```python
from build123d import *

# Parameters (mm, degrees)
SCHIZZO1_W                   = 180
SCHIZZO1_H                   = 60
ESTRUSIONE_ESTRUSIONE1_DEPTH = 5
SCHIZZO1_3_W                 = 180
SCHIZZO1_3_H                 = 10
ESTRUSIONE_ESTRUSIONE2_DEPTH = 100
SCHIZZO2_W                   = 180
SCHIZZO2_H                   = 5
ESTRUSIONE_ESTRUSIONE3_DEPTH = 60
SCHIZZO3_W                   = 5
SCHIZZO3_H                   = 90
ESTRUSIONE_ESTRUSIONE4_DEPTH = 60
SCHIZZO4_W                   = 12
SCHIZZO4_H                   = 3
TAGLIO_ESTRUSIONE1_DEPTH     = 90
SCHIZZO6_W                   = 2
SCHIZZO6_H                   = 15.540639337
ESTRUSIONE_ESTRUSIONE5_DEPTH = 10
SCHIZZO10_W                  = 16
SCHIZZO10_H                  = 3
ESTRUSIONE_ESTRUSIONE7_DEPTH = 30
SCHIZZO11_W                  = 12
SCHIZZO11_H                  = 3
TAGLIO_ESTRUSIONE6_DEPTH     = 5
SCHIZZO12_W                  = 9
SCHIZZO12_H                  = 3
TAGLIO_ESTRUSIONE7_DEPTH     = 20
SCHIZZO13_W                  = 2
SCHIZZO13_H                  = 35.114164676
ESTRUSIONE_ESTRUSIONE8_DEPTH = 10
TAGLIO_ESTRUSIONE8_START     = -15.540639
SCHIZZO15_W                  = 21.926890516
SCHIZZO15_H                  = 11.981890919
TAGLIO_ESTRUSIONE8_DEPTH     = 15.540639
SCHIZZO16_W                  = 12
SCHIZZO16_H                  = 3
ESTRUSIONE_ESTRUSIONE9_DEPTH = 5
SCHIZZO17_R                  = 9.5
TAGLIO_ESTRUSIONE9_DEPTH     = 6
SCHIZZO21_W                  = 2
SCHIZZO21_H                  = 50
TAGLIO_ESTRUSIONE10_DEPTH    = 2


with BuildPart() as part:
    # Schizzo1 → Estrusione-Estrusione1 (new body)
    with BuildSketch(Plane(origin=(0, 0, 0), x_dir=(1, 0, 0), z_dir=(0, 1, 0))):
        with Locations((90, 30)):
            Rectangle(SCHIZZO1_W, SCHIZZO1_H)
    extrude(amount=ESTRUSIONE_ESTRUSIONE1_DEPTH)

    # Schizzo1<3> → Estrusione-Estrusione2 (add)
    with BuildSketch(Plane(origin=(0, 0, 0), x_dir=(1, 0, 0), z_dir=(0, 1, 0))):
        with Locations((90, 65)):
            Rectangle(SCHIZZO1_3_W, SCHIZZO1_3_H)
    extrude(amount=ESTRUSIONE_ESTRUSIONE2_DEPTH)

    # Schizzo2 → Estrusione-Estrusione3 (add)
    with BuildSketch(Plane.XY.offset(-60)):
        with Locations((90, 97.5)):
            Rectangle(SCHIZZO2_W, SCHIZZO2_H)
    extrude(amount=ESTRUSIONE_ESTRUSIONE3_DEPTH)

    # Schizzo3 → Estrusione-Estrusione4 (add)
    with BuildSketch(Plane.XY.offset(-60)):
        with Locations((2.5, 50)):
            Rectangle(SCHIZZO3_W, SCHIZZO3_H)
        with Locations((177.5, 50)):
            Rectangle(SCHIZZO3_W, SCHIZZO3_H)
    extrude(amount=ESTRUSIONE_ESTRUSIONE4_DEPTH)

    # Schizzo4 → Taglio-Estrusione1 (cut)
    with BuildSketch(Plane(origin=(0, 5, 0), x_dir=(1, 0, 0), z_dir=(0, 1, 0))):
        with Locations((50, 40.5)):
            Rectangle(SCHIZZO4_W, SCHIZZO4_H)
    extrude(amount=-TAGLIO_ESTRUSIONE1_DEPTH, mode=Mode.SUBTRACT)

    # Schizzo6 → Estrusione-Estrusione5 (add)
    with BuildSketch(Plane(origin=(0, 5, 0), x_dir=(1, 0, 0), z_dir=(0, 1, 0))):
        with Locations((43, 41.770319669)):
            Rectangle(SCHIZZO6_W, SCHIZZO6_H)
        with Locations((57, 41.770319669)):
            Rectangle(SCHIZZO6_W, SCHIZZO6_H)
    extrude(amount=ESTRUSIONE_ESTRUSIONE5_DEPTH)

    # Schizzo10 → Estrusione-Estrusione7 (add)
    with BuildSketch(Plane.XY.offset(-60)):
        with Locations((50, 33)):
            Rectangle(SCHIZZO10_W, SCHIZZO10_H)
    extrude(amount=ESTRUSIONE_ESTRUSIONE7_DEPTH)

    # Schizzo11 → Taglio-Estrusione6 (cut)
    with BuildSketch(Plane.XZ.offset(-31.5)):
        with Locations((50, -40.5)):
            Rectangle(SCHIZZO11_W, SCHIZZO11_H)
    extrude(amount=-TAGLIO_ESTRUSIONE6_DEPTH, mode=Mode.SUBTRACT)

    # Schizzo12 → Taglio-Estrusione7 (cut)
    with BuildSketch(Plane.XY.offset(-60)):
        with Locations((50, 59)):
            Rectangle(SCHIZZO12_W, SCHIZZO12_H)
    extrude(amount=-TAGLIO_ESTRUSIONE7_DEPTH, mode=Mode.SUBTRACT)

    # Schizzo13 → Estrusione-Estrusione8 (add)
    with BuildSketch(Plane(origin=(0, 34.5, 0), x_dir=(1, 0, 0), z_dir=(0, 1, 0))):
        with Locations((43, 42.442917662)):
            Rectangle(SCHIZZO13_W, SCHIZZO13_H)
        with Locations((57, 42.442917662)):
            Rectangle(SCHIZZO13_W, SCHIZZO13_H)
    extrude(amount=ESTRUSIONE_ESTRUSIONE8_DEPTH)

    # Schizzo15 → Taglio-Estrusione8 (cut)
    with BuildSketch(Plane.XY.offset(-34).offset(TAGLIO_ESTRUSIONE8_START)):
        with Locations((49.332767586, 10.99094546)):
            Rectangle(SCHIZZO15_W, SCHIZZO15_H)
    extrude(amount=TAGLIO_ESTRUSIONE8_DEPTH, mode=Mode.SUBTRACT)

    # Schizzo16 → Estrusione-Estrusione9 (add)
    with BuildSketch(Plane.XZ):
        with Locations((50, -40.5)):
            Rectangle(SCHIZZO16_W, SCHIZZO16_H)
    extrude(amount=-ESTRUSIONE_ESTRUSIONE9_DEPTH)

    # Schizzo17 → Taglio-Estrusione9 (cut)
    with BuildSketch(Plane.XY.offset(-60)):
        with Locations((126, 50.9)):
            Circle(SCHIZZO17_R)
    extrude(amount=-TAGLIO_ESTRUSIONE9_DEPTH, mode=Mode.SUBTRACT)

    # Schizzo21 → Taglio-Estrusione10 (cut)
    with BuildSketch(Plane.XY):
        with Locations((2.5, 50)):
            Rectangle(SCHIZZO21_W, SCHIZZO21_H)
        with Locations((177.5, 50)):
            Rectangle(SCHIZZO21_W, SCHIZZO21_H)
    extrude(amount=-TAGLIO_ESTRUSIONE10_DEPTH, mode=Mode.SUBTRACT)


solid = part.part
```
For this review, take the finished solid that the model builds, in its own axes (mm). A direction names the side the tool comes from. Coordinates: 2 decimals unless noted, no trailing zeros. Write each loop counter-clockwise with the first axis right and the second up, starting at its lowest first coordinate (ties: lowest second). Pieces come first, ordered by that corner, then holes. Notation, with made-up numbers: (66, 69) - (95, 69) arc R5 cw to (95, 78) - close; hole circle Ø11 at (-20.5, 53). An arc over 180 degrees is marked (long way). Put each result on its own line as item: value.
1. For pin 1 (2.5 mm diameter, centred on x = 47.5, y = 32.5, fed in from +Z); pin 2 (1.6 mm diameter, centred on x = 43, y = 40, fed in from +Z); pin 3 (12 mm diameter, centred on x = 113.5, y = 56.5, fed in from +Z), all flat-tipped, find the tip position at first contact; note any pin that passes through.
Values found:
pin 1: z = -30
pin 2: z = -24.89
pin 3: z = -60
2. Add section C-C, the plane y = 62.5. Give the boundary of the cut face in (x, z), then the cut area to 3 significant figures.
Values found:
outline: (0, -70) - (180, -70) - (180, 0) - (178.5, 0) - (178.5, -2) - (176.5, -2) - (176.5, 0) - (175, 0) - (175, -60) - (5, -60) - (5, 0) - (3.5, 0) - (3.5, -2) - (1.5, -2) - (1.5, 0) - (0, 0) - close
area: 2,390 mm²
3. Mouldability with a two-part tool opening along X and no side actions: class faces 4 (the flat face through (175, 49, -30)), 5 (the flat face through (89, 0, -35)), 6 (the flat face through (180, 49, -35)) as released by +X, released by -X, zero draft, split by the parting line, or undercut.
Values found:
face 4: undercut
face 5: zero draft
face 6: released by +X
4. Add section B-B, the plane x = 126. Give the boundary of the cut face in (y, z), then the cut area to 3 significant figures.
Values found:
outline: (0, -70) - (100, -70) - (100, 0) - (95, 0) - (95, -60) - (60.4, -60) - (60.4, -66) - (41.4, -66) - (41.4, -60) - (5, -60) - (5, 0) - (0, 0) - close
area: 1,490 mm²
5. Add section D-D, the plane z = -7.5. Give the boundary of the cut face in (x, y).
Values found:
outline: (0, 0) - (180, 0) - (180, 100) - (0, 100) - close; hole (5, 5) - (175, 5) - (175, 95) - (5, 95) - close
6. Wall thickness on probe 1 along Y at (x, z) = (126, -61); probe 2 along Y at (x, z) = (120.5, -36); probe 3 along X at (y, z) = (54, -6.5): over which ranges is each line inside the solid? List them lowest first.
Values found:
probe 1: 0 to 41.4, 60.4 to 100
probe 2: 0 to 5, 95 to 100
probe 3: 0 to 5, 175 to 180
7. Machinability: for faces 1 (the flat face through (89, 5, -30)), 2 (the flat face through (0, 49, -35)), 3 (the flat face through (50, 57.5, -65)), which of the approach directions +Z, -Z, +X, -X, +Y, -Y give a long, thin tool a straight path to every point of the face, cutting with its end or side? Answer none if there is none.
Values found:
face 1: +Z
face 2: +Z, -Z, -X, +Y, -Y
face 3: +Z, -Z
8. Add section A-A, the plane z = -45. Give the boundary of the cut face in (x, y), then the cut area to 3 significant figures.
Values found:
outline: (0, 0) - (180, 0) - (180, 100) - (0, 100) - close; (42, 31.5) - (58, 31.5) - (58, 44.5) - (56, 44.5) - (56, 34.5) - (44, 34.5) - (44, 44.5) - (42, 44.5) - close; hole (5, 5) - (175, 5) - (175, 95) - (5, 95) - close
area: 2,790 mm²
